```python
from build123d import *

# Parameters (mm, degrees)
F0_W     = 241.3
F0_H     = 38.1
F1_DEPTH = 254
F3_DEPTH = 38.1


with BuildPart() as f1:
    # F0 (on Top) → F1 (new body)
    with BuildSketch(Plane.XY):
        with Locations((10.0588537753, -129.0830521395)):
            Rectangle(F0_W, F0_H)
    extrude(amount=F1_DEPTH)

    # F2 (on face) → F3 (cut)
    with BuildSketch(Plane.XZ.offset(148.1330521395)):
        with BuildLine():
            ThreePointArc((15.302500107, 254), (95.0856852325, 219.171604803), (130.7088537753, 139.7401022129))
            Line((130.7088537753, 139.7401022129), (130.7088537753, 254))
            Line((130.7088537753, 254), (15.302500107, 254))
        make_face()
        with BuildLine():
            ThreePointArc((-110.5911462247, 135.133523386), (-76.4349382663, 217.5345320826), (4.9704818596, 254))
            Line((4.9704818596, 254), (-110.5911462247, 254))
            Line((-110.5911462247, 254), (-110.5911462247, 135.133523386))
        make_face()
    extrude(amount=-F3_DEPTH, mode=Mode.SUBTRACT)


solid = f1.part
```
Can you work these out from the model? Positions are in its coordinate system, mm. Give positions to 0.01 mm unless a question says otherwise; leave off trailing zeros. Write each loop counter-clockwise with the first axis right and the second up, starting at its lowest first coordinate (ties: lowest second). Pieces come first, ordered by that corner, then holes. Notation, with made-up numbers: (-14, 41) -> (27, 41) arc R30 cw to (27, 72) -> close; hole circle Ø2 at (79, 62.5). An arc over 180 degrees is marked (long way). One line per item, written item: value.
Q1. Imagine slicing it at B-B on x = -39.5. Please give me the cut outline in (y, z).
Results found:
outline: (-148.13, 0) -> (-110.03, 0) -> (-110.03, 243.44) -> (-148.13, 243.44) -> close
Q2. Please list where these lines run through material, in increasing order: line 1 (X direction, y = -141, z = 203); line 2 (Z direction, x = 3, y = -137.5); line 3 (X direction, y = -129.5, z = 190). Write a range as [from, to].
Results found:
line 1: x = [-88.5, 108.78]
line 2: z = [0, 253.9]
line 3: x = [-96.5, 116.77]
Q3. Imagine slicing it at A-A on y = -120. Please give me the cut outline in (x, z).
Results found:
outline: (-110.59, 0) -> (130.71, 0) -> (130.71, 139.74) arc R120.74 ccw to (15.3, 254) -> (4.97, 254) arc R120.74 ccw to (-110.59, 135.13) -> close
Q4. Imagine slicing it at C-C on z = 161. Please give me the cut outline in (x, y).
Results found:
outline: (-107.4, -148.13) -> (127.67, -148.13) -> (127.67, -110.03) -> (-107.4, -110.03) -> close
Q5. For P1, Ø1.5, axis at x = -25.5, y = -124, coming from the -Z side; P2, Ø5, axis at x = 61, y = -132, coming from the +Z side, each with a flat end and sliding along its axis, tell me the tip position at first contact or that it passes through.
Results found:
P1: stops at z = 0
P2: stops at z = 244
